from build123d import *
from build123d.topology import SkipClean

# Parameters (mm, degrees)
ESQUISSE1_R             = 75.75
ESQUISSE1_R_2           = 17.15
BOSS_EXTRU_2_DEPTH      = 192
ESQUISSE2_R             = 76
ESQUISSE2_R_2           = 71.5
ENL_V_MAT_EXTRU_1_DEPTH = 310
ESQUISSE3_R             = 75.5
ESQUISSE3_R_2           = 2
BOSS_EXTRU_3_DEPTH      = 5
ESQUISSE4_R             = 2.1
ENL_V_MAT_EXTRU_2_DEPTH = 5
ESQUISSE5_R             = 75.5
ESQUISSE5_R_2           = 65.5
BOSS_EXTRU_4_DEPTH      = 8
ENL_V_START             = -10
ESQUISSE6_R             = 2
ENL_V_MAT_EXTRU_4_DEPTH = 10
ESQUISSE8_R             = 2
ESQUISSE8_R_2           = 2.8
ENL_V_MAT_EXTRU_5_DEPTH = 5.7
ESQUISSE10_R            = 1.5
ESQUISSE10_R_2          = 2
ENL_V_MAT_EXTRU_6_DEPTH = 15
ESQUISSE11_R            = 71.5
ENL_V_MAT_EXTRU_7_DEPTH = 8
ESQUISSE12_W            = 7
ESQUISSE12_H            = 1
ENL_V_MAT_EXTRU_8_DEPTH = 0.5
ESQUISSE13_R            = 2.35
BOSS_EXTRU_6_DEPTH      = 3.5
CHANFREIN1_SIZE         = 1


with BuildPart() as part:
    # Esquisse1 → Boss.-Extru.2 (new body)
    with BuildSketch(Plane.XY):
        Circle(ESQUISSE1_R)
        with Locations((-34.305739626, 47.199986533)):
            Circle(ESQUISSE1_R_2, mode=Mode.SUBTRACT)
        with Locations((-0.010470369, 58.349999061)):
            Circle(ESQUISSE1_R_2, mode=Mode.SUBTRACT)
        with Locations((34.288798212, 47.212295191)):
            Circle(ESQUISSE1_R_2, mode=Mode.SUBTRACT)
        with Locations((55.49091131, 18.041099245)):
            Circle(ESQUISSE1_R_2, mode=Mode.SUBTRACT)
        with Locations((55.497382355, -18.021183418)):
            Circle(ESQUISSE1_R_2, mode=Mode.SUBTRACT)
        with Locations((34.305739626, -47.199986533)):
            Circle(ESQUISSE1_R_2, mode=Mode.SUBTRACT)
        with Locations((0.010470369, -58.349999061)):
            Circle(ESQUISSE1_R_2, mode=Mode.SUBTRACT)
        with Locations((-34.288798212, -47.212295191)):
            Circle(ESQUISSE1_R_2, mode=Mode.SUBTRACT)
        with Locations((-55.49091131, -18.041099245)):
            Circle(ESQUISSE1_R_2, mode=Mode.SUBTRACT)
        with Locations((-55.497382355, 18.021183418)):
            Circle(ESQUISSE1_R_2, mode=Mode.SUBTRACT)
        with Locations((-21.759702771, 11.082204515)):
            Circle(ESQUISSE1_R_2, mode=Mode.SUBTRACT)
        with Locations((11.082204515, 21.759702771)):
            Circle(ESQUISSE1_R_2, mode=Mode.SUBTRACT)
        with Locations((21.759702771, -11.082204515)):
            Circle(ESQUISSE1_R_2, mode=Mode.SUBTRACT)
        with Locations((-11.082204515, -21.759702771)):
            Circle(ESQUISSE1_R_2, mode=Mode.SUBTRACT)
    extrude(amount=BOSS_EXTRU_2_DEPTH)

    # Esquisse2 → Enlèv. mat.-Extru.1 (cut)
    with BuildSketch(Plane(origin=(0, 0, 0), x_dir=(-1, 0, 0), z_dir=(0, 0, -1))):
        Circle(ESQUISSE2_R)
        Circle(ESQUISSE2_R_2, mode=Mode.SUBTRACT)
    extrude(amount=-ENL_V_MAT_EXTRU_1_DEPTH, mode=Mode.SUBTRACT)

    # Esquisse3 → Boss.-Extru.3 (add)
    with BuildSketch(Plane(origin=(0, 0, 0), x_dir=(-1, 0, 0), z_dir=(0, 0, -1))):
        Circle(ESQUISSE3_R)
        with Locations((6.776911329, -64.589491695)):
            Circle(ESQUISSE3_R_2, mode=Mode.SUBTRACT)
        with Locations((-6.788589165, 64.700790989)):
            Circle(ESQUISSE3_R_2, mode=Mode.SUBTRACT)
    extrude(amount=BOSS_EXTRU_3_DEPTH)

    # Esquisse4 → Enlèv. mat.-Extru.2 (cut)
    with BuildSketch(Plane(origin=(0, 0, -5), x_dir=(-1, 0, 0), z_dir=(0, 0, -1))):
        with Locations((55.49091131, -18.041099245)):
            Circle(ESQUISSE4_R)
        with Locations((34.288798212, -47.212295191)):
            Circle(ESQUISSE4_R)
        with Locations((-0.010470369, -58.349999061)):
            Circle(ESQUISSE4_R)
        with Locations((-34.305739626, -47.199986533)):
            Circle(ESQUISSE4_R)
        with Locations((-55.497382355, -18.021183418)):
            Circle(ESQUISSE4_R)
        with Locations((-55.49091131, 18.041099245)):
            Circle(ESQUISSE4_R)
        with Locations((-34.288798212, 47.212295191)):
            Circle(ESQUISSE4_R)
        with Locations((0.010470369, 58.349999061)):
            Circle(ESQUISSE4_R)
        with Locations((34.305739626, 47.199986533)):
            Circle(ESQUISSE4_R)
        with Locations((55.497382355, 18.021183418)):
            Circle(ESQUISSE4_R)
        with Locations((11.082204515, -21.759702771)):
            Circle(ESQUISSE4_R)
        with Locations((-21.759702771, -11.082204515)):
            Circle(ESQUISSE4_R)
        with Locations((-11.082204515, 21.759702771)):
            Circle(ESQUISSE4_R)
        with Locations((21.759702771, 11.082204515)):
            Circle(ESQUISSE4_R)
    extrude(amount=-ENL_V_MAT_EXTRU_2_DEPTH, mode=Mode.SUBTRACT)

    # Esquisse5 → Boss.-Extru.4 (add)
    with BuildSketch(Plane(origin=(0, 0, -5), x_dir=(-1, 0, 0), z_dir=(0, 0, -1))):
        Circle(ESQUISSE5_R)
        with Locations(Location((0, 0, 0), (0, 0, 97.701419097))):
            Circle(ESQUISSE5_R_2, mode=Mode.SUBTRACT)
    extrude(amount=BOSS_EXTRU_4_DEPTH)

    # Esquisse6 → Enlèv. mat.-Extru.4 (cut)
    with SkipClean():  # the faces are left unmerged after this step: merging them gives an invalid solid
        with BuildSketch(Plane(origin=(0, 0, -13), x_dir=(-1, 0, 0), z_dir=(0, 0, -1)).offset(ENL_V_START)):
            with Locations(Location((-6.788589165, 64.700790989, 0), (0, 0, 174.019176169))):
                Circle(ESQUISSE6_R)
            with Locations(Location((6.776911329, -64.589491695, 0), (0, 0, 201.283568474))):
                Circle(ESQUISSE6_R)
        extrude(amount=ENL_V_MAT_EXTRU_4_DEPTH, mode=Mode.SUBTRACT)
    add(part.part.scale(1), mode=Mode.REPLACE)  # the faces are merged on a copy

    # Esquisse8 → Enlèv. mat.-Extru.5 (cut)
    with BuildSketch(Plane.XY.offset(192)):
        with Locations((-20.704138623, -63.720786592)):
            Circle(ESQUISSE8_R)
        with Locations((-67, 0)):
            Circle(ESQUISSE8_R)
        with Locations((-20.704138623, 63.720786592)):
            Circle(ESQUISSE8_R)
        with Locations((54.204138623, 39.381611904)):
            Circle(ESQUISSE8_R)
        with Locations((54.204138623, -39.381611904)):
            Circle(ESQUISSE8_R)
        Circle(ESQUISSE8_R_2)
    extrude(amount=-ENL_V_MAT_EXTRU_5_DEPTH, mode=Mode.SUBTRACT)

    # Esquisse10 → Enlèv. mat.-Extru.6 (cut)
    with BuildSketch(Plane.XY.offset(186.3)):
        with Locations((-20.704138623, -63.720786592)):
            Circle(ESQUISSE10_R)
        with Locations((-67, 0)):
            Circle(ESQUISSE10_R)
        with Locations((-20.704138623, 63.720786592)):
            Circle(ESQUISSE10_R)
        with Locations((54.204138623, 39.381611904)):
            Circle(ESQUISSE10_R)
        with Locations((54.204138623, -39.381611904)):
            Circle(ESQUISSE10_R)
        Circle(ESQUISSE10_R_2)
    extrude(amount=-ENL_V_MAT_EXTRU_6_DEPTH, mode=Mode.SUBTRACT)

    # Esquisse11 → Enlèv. mat.-Extru.7 (cut)
    with BuildSketch(Plane(origin=(0, 0, -13), x_dir=(-1, 0, 0), z_dir=(0, 0, -1))):
        Circle(ESQUISSE11_R)
    extrude(amount=-ENL_V_MAT_EXTRU_7_DEPTH, mode=Mode.SUBTRACT)

    # Esquisse12 → Enlèv. mat.-Extru.8 (cut)
    with BuildSketch(Plane.XY):
        with Locations((0.010470369, -69.659338912)):
            Rectangle(ESQUISSE12_W, ESQUISSE12_H)
        Polygon((-0.510470369, 70.811208438), (-0.510470369, 73.811208438), (0.489529631, 73.811208438), (0.489529631, 70.811208438), (3.489529631, 70.811208438), (3.489529631, 69.811208438), (0.489529631, 69.811208438), (0.489529631, 66.811208438), (-0.510470369, 66.811208438), (-0.510470369, 69.811208438), (-3.510470369, 69.811208438), (-3.510470369, 70.811208438), align=None)
    extrude(amount=-ENL_V_MAT_EXTRU_8_DEPTH, mode=Mode.SUBTRACT)

    # Esquisse13 → Boss.-Extru.6 (add)
    with BuildSketch(Plane.XY.offset(192)):
        with Locations((67, 0)):
            Circle(ESQUISSE13_R)
    extrude(amount=BOSS_EXTRU_6_DEPTH)

    # Chanfrein1
    chanfrein1_edges = [part.edges().sort_by_distance(p)[0] for p in [
        (64.65, 0, 195.5),
    ]]
    chamfer(chanfrein1_edges, length=CHANFREIN1_SIZE)


solid = part.part
Could you check a few things on this model? Use its own coordinates, in mm. A direction names the side the tool comes from. Give positions to 0.01 mm unless a question says otherwise; leave off trailing zeros. Order: outer loops, then holes, each group sorted by start corner. A loop starts at its lowest first (then second) coordinate and runs counter-clockwise, first axis right, second up. Notation, with made-up numbers: (71, 34.25) - (103, 34.25) arc R26 ccw to (103, 68.25) - close; hole circle Ø7 at (-28, 35). An arc over 180 degrees is marked (long way). Return JSON: item names as keys, results as strings. Group by question number.
Q1. Thinking about a two-plate mould opening in Y: for faces 4 (the face through (71.5, 0.2, 94.7)), 5 (the face through (57.937, -41.9, 94.656)), 6 (the face through (45, -56, -13)), 7 (the face through (5.276, -16.608, 94.656)), which applies, pulls with the +Y half, pulls with the -Y half, needs draft (parallel to the pull), parting line crosses it, or undercut?
Q2. Will these pins go through, and if not, where does the flat tip stop? pin 1 Ø2 at (y, z) = (-35.5, 155.5) entering from +X; pin 2 Ø1.5 at (x, z) = (-31, 59.5) entering from -Y; pin 3 Ø5 at (x, y) = (-6.78, -64.59) entering from +Z; pin 4 Ø3.5 at (x, y) = (-0.01, 58.35) entering from -Z.
Q3. Please list where these lines run through material, in increasing order: line 1 along X through (y, z) = (2.5, 185); line 2 along X through (y, z) = (46.5, 110); line 3 along X through (y, z) = (-18, 106). Write a range as [from, to].
Q4. Which directions (+Z, -Z, +X, -X, +Y, -Y) give clear straight access to the entire face, cutting with the end or side of a thin tool? Please do faces 1 (the face through (22.243, -67.952, 94.656)), 2 (the face through (-0.57, 41.21, 94.66)), 3 (the face through (-21.946, -68.049, 94.656)).
Q5. Suppose I cut it at A-A, the plane z = 93. Please give me the cut outline in (x, y), and give its area (3 significant figures).
Resolved:
{
 "1": {"face 4": "parting line crosses it", "face 5": "pulls with the -Y half", "face 6": "needs draft", "face 7": "undercut"},
 "2": {"pin 1": "stops at x = 62.63", "pin 2": "stops at y = -64.79", "pin 3": "stops at z = 0", "pin 4": "passes through"},
 "3": {"line 1": "x = [-71.46, -62.79], [-48.2, -36.61], [-6.91, 11.29], [32.23, 48.24], [62.74, 71.46]", "line 2": "x = [-54.31, -51.44], [-17.17, -12.41], [12.39, 17.15], [51.42, 54.31]", "line 3": "x = [-38.34, -27.82], [5.65, 6.07], [37.45, 38.35]"},
 "4": {"face 1": "+Z, +X, -Y", "face 2": "+Z", "face 3": "+Z, -X, -Y"},
 "5": {"outline": "(-70.77, 10.21) arc R71.5 ccw to (-70.76, -10.24) arc R17.15 cw (long way) to (-63.25, -33.33) arc R71.5 ccw to (-51.23, -49.88) arc R17.15 cw (long way) to (-31.58, -64.15) arc R71.5 ccw to (-12.13, -70.46) arc R17.15 cw (long way) to (12.15, -70.46) arc R71.5 ccw to (31.6, -64.14) arc R17.15 cw (long way) to (51.25, -49.86) arc R71.5 ccw to (63.27, -33.31) arc R17.15 cw (long way) to (70.77, -10.21) arc R71.5 ccw to (70.76, 10.24) arc R17.15 cw (long way) to (63.25, 33.33) arc R71.5 ccw to (51.23, 49.88) arc R17.15 cw (long way) to (31.58, 64.15) arc R71.5 ccw to (12.13, 70.46) arc R17.15 cw (long way) to (-12.15, 70.46) arc R71.5 ccw to (-31.6, 64.14) arc R17.15 cw (long way) to (-51.25, 49.86) arc R71.5 ccw to (-63.27, 33.31) arc R17.15 cw (long way) to start; hole circle Ø34.3 at (-21.76, 11.08); hole circle Ø34.3 at (-11.08, -21.76); hole circle Ø34.3 at (11.08, 21.76); hole circle Ø34.3 at (21.76, -11.08)", "area": "3,800 mm2"}
}
